```python
from build123d import *

# Parameters (mm, degrees)
BOSS_EXTRUDE1_DEPTH = 4
CUT_EXTRUDE1_DEPTH  = 10


with BuildPart() as part:
    # Sketch1 → Boss-Extrude1 (new body)
    with BuildSketch(Plane(origin=(0, 0, 0), x_dir=(1, 0, 0), z_dir=(0, 1, 0))):
        Polygon((-17.714285714, -48), (-17.714285714, -58), (78.285714286, -58), (78.285714286, -48), (82.285714286, -48), (82.285714286, -44), (78.285714286, -44), (78.285714286, -32), (82.285714286, -32), (82.285714286, -28), (78.285714286, -28), (78.285714286, -16), (82.285714286, -16), (82.285714286, -12), (78.285714286, -12), (78.285714286, 0), (82.285714286, 0), (82.285714286, 4), (78.285714286, 4), (78.285714286, 14), (-17.714285714, 14), (-17.714285714, 4), (-21.714285714, 4), (-21.714285714, 0), (-17.714285714, 0), (-17.714285714, -12), (-21.714285714, -12), (-21.714285714, -16), (-17.714285714, -16), (-17.714285714, -28), (-21.714285714, -28), (-21.714285714, -32), (-17.714285714, -32), (-17.714285714, -44), (-21.714285714, -44), (-21.714285714, -48), align=None)
    extrude(amount=-BOSS_EXTRUDE1_DEPTH)

    # Sketch2 → Cut-Extrude1 (cut)
    with BuildSketch(Plane(origin=(0, 0, 0), x_dir=(1, 0, 0), z_dir=(0, 1, 0))):
        with BuildLine():
            ThreePointArc((-13.714285714, 2.94278394), (-12.661123549, 4.704458744), (-10.6107876, 4.610804297))
            Line((-10.6107876, 4.610804297), (19.53422954, -15.331979643))
            ThreePointArc((19.53422954, -15.331979643), (20.345939079, -17.576176746), (18.430731426, -19))
            Line((18.430731426, -19), (-11.714285714, -19))
            ThreePointArc((-11.714285714, -19), (-13.128499277, -18.414213562), (-13.714285714, -17))
            Line((-13.714285714, -17), (-13.714285714, 2.94278394))
        make_face()
        with BuildLine():
            Line((-4.859302854, 10), (25.285714286, 10))
            ThreePointArc((25.285714286, 10), (26.699927848, 9.414213562), (27.285714286, 8))
            Line((27.285714286, 8), (27.285714286, -11.94278394))
            ThreePointArc((27.285714286, -11.94278394), (26.23255212, -13.704458744), (24.182216171, -13.610804297))
            Line((24.182216171, -13.610804297), (-5.962800969, 6.331979643))
            ThreePointArc((-5.962800969, 6.331979643), (-6.774510508, 8.576176746), (-4.859302854, 10))
        make_face()
        with BuildLine():
            Line((33.285714286, 8), (33.285714286, -11.94278394))
            ThreePointArc((33.285714286, -11.94278394), (34.338876451, -13.704458744), (36.3892124, -13.610804297))
            Line((36.3892124, -13.610804297), (66.53422954, 6.331979643))
            ThreePointArc((66.53422954, 6.331979643), (67.345939079, 8.576176746), (65.430731426, 10))
            Line((65.430731426, 10), (35.285714286, 10))
            ThreePointArc((35.285714286, 10), (33.871500723, 9.414213562), (33.285714286, 8))
        make_face()
        with BuildLine():
            ThreePointArc((74.285714286, -17), (73.699927848, -18.414213562), (72.285714286, -19))
            Line((72.285714286, -19), (42.140697146, -19))
            ThreePointArc((42.140697146, -19), (40.225489492, -17.576176746), (41.037199031, -15.331979643))
            Line((41.037199031, -15.331979643), (71.182216171, 4.610804297))
            ThreePointArc((71.182216171, 4.610804297), (73.23255212, 4.704458744), (74.285714286, 2.94278394))
            Line((74.285714286, 2.94278394), (74.285714286, -17))
        make_face()
        with BuildLine():
            ThreePointArc((74.285714286, -46.94278394), (73.23255212, -48.704458744), (71.182216171, -48.610804297))
            Line((71.182216171, -48.610804297), (41.037199031, -28.668020357))
            ThreePointArc((41.037199031, -28.668020357), (40.225489492, -26.423823254), (42.140697146, -25))
            Line((42.140697146, -25), (72.285714286, -25))
            ThreePointArc((72.285714286, -25), (73.699927848, -25.585786438), (74.285714286, -27))
            Line((74.285714286, -27), (74.285714286, -46.94278394))
        make_face()
        with BuildLine():
            Line((65.430731426, -54), (35.285714286, -54))
            ThreePointArc((35.285714286, -54), (33.871500723, -53.414213562), (33.285714286, -52))
            Line((33.285714286, -52), (33.285714286, -32.05721606))
            ThreePointArc((33.285714286, -32.05721606), (34.338876451, -30.295541256), (36.3892124, -30.389195703))
            Line((36.3892124, -30.389195703), (66.53422954, -50.331979643))
            ThreePointArc((66.53422954, -50.331979643), (67.345939079, -52.576176746), (65.430731426, -54))
        make_face()
        with BuildLine():
            Line((27.285714286, -52), (27.285714286, -32.05721606))
            ThreePointArc((27.285714286, -32.05721606), (26.23255212, -30.295541256), (24.182216171, -30.389195703))
            Line((24.182216171, -30.389195703), (-5.962800969, -50.331979643))
            ThreePointArc((-5.962800969, -50.331979643), (-6.774510508, -52.576176746), (-4.859302854, -54))
            Line((-4.859302854, -54), (25.285714286, -54))
            ThreePointArc((25.285714286, -54), (26.699927848, -53.414213562), (27.285714286, -52))
        make_face()
        with BuildLine():
            ThreePointArc((-13.714285714, -27), (-13.128499277, -25.585786438), (-11.714285714, -25))
            Line((-11.714285714, -25), (18.430731426, -25))
            ThreePointArc((18.430731426, -25), (20.345939079, -26.423823254), (19.53422954, -28.668020357))
            Line((19.53422954, -28.668020357), (-10.6107876, -48.610804297))
            ThreePointArc((-10.6107876, -48.610804297), (-12.661123549, -48.704458744), (-13.714285714, -46.94278394))
            Line((-13.714285714, -46.94278394), (-13.714285714, -27))
        make_face()
    extrude(amount=-CUT_EXTRUDE1_DEPTH, mode=Mode.SUBTRACT)


solid = part.part
```
For this review, take the finished solid that the model builds, in its own axes (mm). A direction names the side the tool comes from. Round coordinates to 2 decimals unless told otherwise and drop trailing zeros. Write each loop counter-clockwise with the first axis right and the second up, starting at its lowest first coordinate (ties: lowest second). Pieces come first, ordered by that corner, then holes. Notation, with made-up numbers: (-26, 16.5) - (-4, 16.5) arc R8 ccw to (-4, 28.5) - close; hole circle Ø3 at (6.5, 1.25). An arc over 180 degrees is marked (long way). Answer as a JSON object with one key per item and string values.
1. To check wall thickness, follow line 1 along Z through (x, y) = (25.5, -0.3); line 2 along X through (y, z) = (-2.8, 52); line 3 along Z through (x, y) = (6, -0.45). State the ranges of each line that lie inside material, in increasing order.
Response values:
{"line 1": "z = -14 to -9.99, 13.93 to 30.07, 53.99 to 58", "line 2": "x = -17.71 to -6.86, 27.29 to 33.29, 67.43 to 78.29", "line 3": "z = -14 to -10, 1.58 to 6.38, 19 to 25, 37.62 to 42.42, 54 to 58"}
2. We need section C-C on x = 55.5. Give the boundary of the cut face in (y, z).
Response values:
{"outline": "(-4, -14) - (0, -14) - (0, -10) - (-4, -10) - close; (-4, 0.97) - (0, 0.97) - (0, 5.76) - (-4, 5.76) - close; (-4, 19) - (0, 19) - (0, 25) - (-4, 25) - close; (-4, 38.24) - (0, 38.24) - (0, 43.03) - (-4, 43.03) - close; (-4, 54) - (0, 54) - (0, 58) - (-4, 58) - close"}
3. Draft analysis for pull direction X (two halves, no side actions). For faces 5 (the face through (-21.714, -2, -2)), 6 (the face through (30, -4, 13)), 7 (the face through (33.286, -2, 42)), 8 (the face through (82.286, -2, -2)), state which applies: +X half, -X half, draft (parallel to the pull), parting line (faces both ways), or undercut.
Response values:
{"face 5": "-X half", "face 6": "draft", "face 7": "undercut", "face 8": "+X half"}
4. We need section A-A on x = -8. Give the boundary of the cut face in (y, z).
Response values:
{"outline": "(-4, -14) - (0, -14) - (0, -2.88) - (-4, -2.88) - close; (-4, 19) - (0, 19) - (0, 25) - (-4, 25) - close; (-4, 46.88) - (0, 46.88) - (0, 58) - (-4, 58) - close"}
5. Tool access review of faces 1 (the face through (80, -2, -4)), 2 (the face through (-20, -2, 16)), 3 (the face through (-20, -2, 48)), 4 (the face through (26.26, -1.97, 30.31)): name each direction out of +Z, -Z, +X, -X, +Y, -Y from which nothing blocks a thin tool from reaching the whole face with its end or side.
Response values:
{"face 1": "-Z, +X, +Y, -Y", "face 2": "-X, +Y, -Y", "face 3": "+Z, -X, +Y, -Y", "face 4": "+Y, -Y"}
6. For pin 1 Ø2 at (x, y) = (81, -2) entering from +Z; pin 2 Ø1 at (y, z) = (-3, 2) entering from +X, all flat-tipped, find the tip position at first contact; note any pin that passes through.
Response values:
{"pin 1": "stops at z = 48", "pin 2": "stops at x = 78.29"}
7. We need section D-D on y = -2.65. Count the separate pieces of the cut face and the enclosed holes in it, then the cut area to 3 significant figures.
Response values:
{"separate pieces": "1", "enclosed holes": "8", "area": "3,160 mm2"}
8. We need section B-B on z = 37.5. Give the boundary of the cut face in (x, y), then the cut area to 3 significant figures.
Response values:
{"outline": "(-17.71, -4) - (-13.71, -4) - (-13.71, 0) - (-17.71, 0) - close; (6.18, -4) - (13.43, -4) - (13.43, 0) - (6.18, 0) - close; (27.29, -4) - (33.29, -4) - (33.29, 0) - (27.29, 0) - close; (47.14, -4) - (54.39, -4) - (54.39, 0) - (47.14, 0) - close; (74.29, -4) - (78.29, -4) - (78.29, 0) - (74.29, 0) - close", "area": "114 mm2"}
